Design review of the part built by this model. Coordinates are the model's own, in mm. Face numbers are marked on the shaded views. A direction names the side the tool comes from. Coordinates: 2 decimals unless noted, no trailing zeros. Write each loop counter-clockwise with the first axis right and the second up, starting at its lowest first coordinate (ties: lowest second). Pieces come first, ordered by that corner, then holes. Notation, with made-up numbers: M -18.5,28.5 L 6.5,28.5 A12 cw 6.5,42.5 Z; hole C 25,34 d8. An arc over 180 degrees is marked long. Return JSON: item names as keys, results as strings. Group by question number.
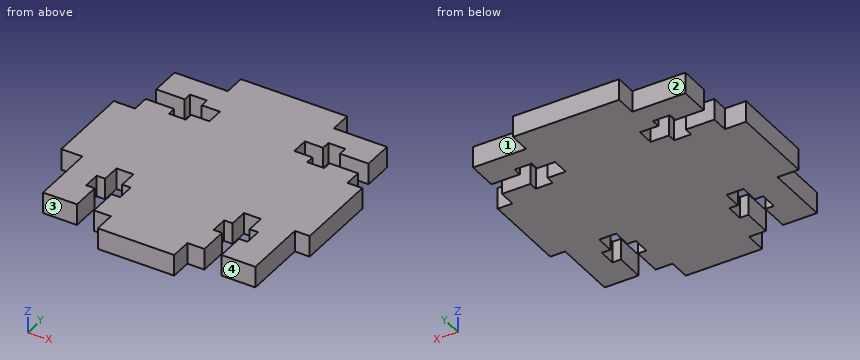
Autodesk Inventor part; units mm, degrees
ref_plane "YZ Plane" through (0, 0, 0) normal (1, 0, 0) x (0, 1, 0)
ref_plane "XZ Plane" through (0, 0, 0) normal (0, 1, 0) x (-1, 0, 0)
ref_plane "XY Plane" through (0, 0, 0) normal (0, 0, 1) x (1, 0, 0)
sketch "Sketch1" plane through (0, 0, 0) normal (0, 0, 1) x (1, 0, 0)
  line L0 (-25, -25) -> (25, -25)
  line L1 (25, -25) -> (25, 25)
  line L2 (25, 25) -> (-25, 25)
  line L3 (-25, 25) -> (-25, -25)
  line L4 (-25, -25) -> (25, 25) construction
  line L5 (25, -25) -> (-25, 25) construction
  point P0 (0, 0)
  dimension "d0" = 50
  dimension "d1" = 50
extrude "Extrusion1" add sketch "Sketch1" along normal blind 5
sketch "Sketch2" plane through (0, 0, 5) normal (0, 0, 1) x (1, 0, 0)
  line L0 (-25, -25) -> (25, -25) construction
  line L1 (25, -25) -> (25, 25) construction
  line L2 (25, 25) -> (-25, 25) construction
  line L3 (-25, 25) -> (-25, -25) construction
  line L4 (-25, -25) -> (25, -25) construction
  line L5 (-9, -25) -> (9, -25)
  line L6 (9, -25) -> (9, -30)
  line L7 (9, -30) -> (-9, -30)
  line L8 (-9, -30) -> (-9, -25)
  line L9 (-25, 10) -> (-30, 10)
  line L10 (-30, 10) -> (-30, -10)
  line L11 (-30, -10) -> (-25, -10)
  line L12 (-25, -10) -> (-25, 10)
  line L13 (25, 25) -> (-25, 25) construction
  line L14 (-12.5, 25) -> (12.5, 25)
  line L15 (12.5, 25) -> (12.5, 30)
  line L16 (12.5, 30) -> (-12.5, 30)
  line L17 (-12.5, 30) -> (-12.5, 25)
  line L18 (25, -10) -> (28.5, -10)
  line L19 (28.5, -10) -> (28.5, 10)
  line L20 (28.5, 10) -> (25, 10)
  line L21 (25, 10) -> (25, -10)
  point P0 (0, 0)
  dimension "d4" = 18
  dimension "d5" = 5
  dimension "d6" = 16
  dimension "d7" = 5
  dimension "d8" = 20
  dimension "d9" = 15
  dimension "d10" = 25
  dimension "d11" = 12.5
  dimension "d14" = 3.5
  dimension "d15" = 20
  dimension "d16" = 15
  dimension "d39" = 5
extrude "Extrusion2" add sketch "Sketch2" against normal blind 5
sketch "Sketch3" plane through (0, 0, 5) normal (0, 0, 1) x (1, 0, 0)
  line L0 (-25, -25) -> (-9, -25) construction
  line L1 (-9, -30) -> (-9, -25) construction
  line L2 (9, -30) -> (-9, -30) construction
  line L3 (9, -25) -> (9, -30) construction
  line L4 (9, -25) -> (25, -25) construction
  line L5 (25, -25) -> (25, -10) construction
  line L6 (25, -10) -> (28.5, -10) construction
  line L7 (28.5, -10) -> (28.5, 10) construction
  line L8 (28.5, 10) -> (25, 10) construction
  line L9 (25, 10) -> (25, 25) construction
  line L10 (25, 25) -> (12.5, 25) construction
  line L11 (12.5, 25) -> (12.5, 30) construction
  line L12 (12.5, 30) -> (-12.5, 30) construction
  line L13 (-12.5, 30) -> (-12.5, 25) construction
  line L14 (-12.5, 25) -> (-25, 25) construction
  line L15 (-25, 25) -> (-25, 10) construction
  line L16 (-25, 10) -> (-30, 10) construction
  line L17 (-30, 10) -> (-30, -10) construction
  line L18 (-30, -10) -> (-25, -10) construction
  line L19 (-25, -10) -> (-25, -25) construction
  line L20 (-25, 25) -> (-25, 10) construction
  line L21 (-25, 18) -> (-10, 18) construction
  line L22 (-10, 18) -> (-10, 14) construction
  line L23 (-10, 14) -> (-25, 14) construction
  line L24 (-25, 14) -> (-25, 18) construction
  line L25 (-10, 16) -> (-25, 16) construction
  line L26 (-18.2831, 12) -> (-14.2831, 12) construction
  line L27 (-14.2831, 12) -> (-14.2831, 20) construction
  line L28 (-14.2831, 20) -> (-18.2831, 20) construction
  line L29 (-18.2831, 20) -> (-18.2831, 12) construction
  line L30 (-18.2831, 12) -> (-14.2831, 20) construction
  line L31 (-14.2831, 12) -> (-18.2831, 20) construction
  line L32 (-25, 14) -> (-25, 18)
  line L33 (-25, 18) -> (-18.2831, 18)
  line L34 (-18.2831, 18) -> (-18.2831, 20)
  line L35 (-18.2831, 20) -> (-14.2831, 20)
  line L36 (-14.2831, 20) -> (-14.2831, 18)
  line L37 (-14.2831, 18) -> (-10, 18)
  line L38 (-10, 18) -> (-10, 14)
  line L39 (-10, 14) -> (-14.2831, 14)
  line L40 (-14.2831, 14) -> (-14.2831, 12)
  line L41 (-14.2831, 12) -> (-18.2831, 12)
  line L42 (-18.2831, 12) -> (-18.2831, 14)
  line L43 (-18.2831, 14) -> (-25, 14)
  line L44 (-17, -25) -> (-17, -10) construction
  line L45 (-17, -10) -> (-13, -10) construction
  line L46 (-13, -10) -> (-13, -25) construction
  line L47 (-13, -25) -> (-17, -25) construction
  line L48 (-15, -10) -> (-15, -25) construction
  line L49 (-11, -18.2831) -> (-11, -14.2831) construction
  line L50 (-11, -14.2831) -> (-19, -14.2831) construction
  line L51 (-19, -14.2831) -> (-19, -18.2831) construction
  line L52 (-19, -18.2831) -> (-11, -18.2831) construction
  line L53 (-11, -18.2831) -> (-19, -14.2831) construction
  line L54 (-11, -14.2831) -> (-19, -18.2831) construction
  line L55 (-13, -25) -> (-17, -25)
  line L56 (-17, -25) -> (-17, -18.2831)
  line L57 (-17, -18.2831) -> (-19, -18.2831)
  line L58 (-19, -18.2831) -> (-19, -14.2831)
  line L59 (-19, -14.2831) -> (-17, -14.2831)
  line L60 (-17, -14.2831) -> (-17, -10)
  line L61 (-17, -10) -> (-13, -10)
  line L62 (-13, -10) -> (-13, -14.2831)
  line L63 (-13, -14.2831) -> (-11, -14.2831)
  line L64 (-11, -14.2831) -> (-11, -18.2831)
  line L65 (-11, -18.2831) -> (-13, -18.2831)
  line L66 (-13, -18.2831) -> (-13, -25)
  line L67 (13, -10) -> (17, -10) construction
  line L68 (13, -10) -> (17, -10)
  line L69 (11, -14.2831) -> (13, -14.2831)
  line L70 (13, -14.2831) -> (13, -10)
  line L71 (17, -10) -> (17, -14.2831)
  line L72 (19, -14.2831) -> (11, -14.2831) construction
  line L73 (17, -14.2831) -> (19, -14.2831)
  line L74 (11, -14.2831) -> (11, -18.2831) construction
  line L75 (11, -18.2831) -> (11, -14.2831)
  line L76 (19, -18.2831) -> (11, -14.2831) construction
  line L77 (19, -14.2831) -> (11, -18.2831) construction
  line L78 (19, -18.2831) -> (19, -14.2831) construction
  line L79 (19, -14.2831) -> (19, -18.2831)
  line L80 (13, -25) -> (13, -10) construction
  line L81 (15, -10) -> (15, -25) construction
  line L82 (17, -10) -> (17, -25) construction
  line L83 (13, -18.2831) -> (11, -18.2831)
  line L84 (19, -18.2831) -> (17, -18.2831)
  line L85 (17, -18.2831) -> (17, -25)
  line L86 (17, -25) -> (13, -25) construction
  line L87 (17, -25) -> (13, -25)
  line L88 (13, -25) -> (13, -18.2831)
  line L89 (11, -18.2831) -> (19, -18.2831) construction
  line L90 (25, 14) -> (10, 14) construction
  line L91 (10, 14) -> (10, 18) construction
  line L92 (10, 18) -> (25, 18) construction
  line L93 (25, 18) -> (25, 14) construction
  line L94 (10, 16) -> (25, 16) construction
  line L95 (18.2831, 20) -> (14.2831, 20) construction
  line L96 (14.2831, 20) -> (14.2831, 12) construction
  line L97 (14.2831, 12) -> (18.2831, 12) construction
  line L98 (18.2831, 12) -> (18.2831, 20) construction
  line L99 (18.2831, 20) -> (14.2831, 12) construction
  line L100 (14.2831, 20) -> (18.2831, 12) construction
  line L101 (25, 18) -> (25, 14)
  line L102 (25, 14) -> (18.2831, 14)
  line L103 (18.2831, 14) -> (18.2831, 12)
  line L104 (18.2831, 12) -> (14.2831, 12)
  line L105 (14.2831, 12) -> (14.2831, 14)
  line L106 (14.2831, 14) -> (10, 14)
  line L107 (10, 14) -> (10, 18)
  line L108 (10, 18) -> (14.2831, 18)
  line L109 (14.2831, 18) -> (14.2831, 20)
  line L110 (14.2831, 20) -> (18.2831, 20)
  line L111 (18.2831, 20) -> (18.2831, 18)
  line L112 (18.2831, 18) -> (25, 18)
  point P0 (0, 0)
  point P1 (-16.2831, 16)
  point P2 (-15, -16.2831)
  point P3 (15, -16.2831)
  point P4 (16.2831, 16)
  dimension "d17" = 15
  dimension "d18" = 4
  dimension "d19" = 4
  dimension "d20" = 8
  dimension "d21" = 15
  dimension "d22" = 4
  dimension "d23" = 4
  dimension "d24" = 8
  dimension "d25" = 15
  dimension "d26" = 4
  dimension "d27" = 4
  dimension "d28" = 8
  dimension "d29" = 8
  dimension "d30" = 4
  dimension "d31" = 4
  dimension "d32" = 15
  dimension "d33" = 4
  dimension "d34" = 4
  dimension "d35" = 8
  dimension "d36" = 7
extrude "Extrusion3" cut sketch "Sketch3" against normal blind 5
properties part number "Soporte_Ducto_Rod"
Item 1: Add section A-A (y = 13). Write out the cut boundary in (x, z).
Item 2: For pin 1 (1 mm diameter, centred on x = 18, z = 3, fed in from +Y); pin 2 (0.6 mm diameter, centred on x = 18, z = 2, fed in from -Y); pin 3 (1.6 mm diameter, centred on y = 12.5, z = 1.5, fed in from +X), all flat-tipped, find the tip position at first contact; note any pin that passes through.
Item 3: For line 1 (X direction, y = -11, z = 4.35); line 2 (Y direction, x = 18.5, z = 4.2); line 3 (Y direction, x = 21.5, z = 0.2), list the stretches that pass through material, from the lowest coordinate up.
Item 4: Add section B-B (y = -17). Write out the cut boundary in (x, z).
Item 5: Machinability: for the marked faces 1, 2, 3 and 4, which of the approach directions +Z, -Z, +X, -X, +Y, -Y give a long, thin tool a straight path to every point of the face, cutting with its end or side? Answer none if there is none.
Geometry check:
{
 "1": {"outline": "M -25,0 L -18.28,0 L -18.28,5 L -25,5 Z; M -14.28,0 L 14.28,0 L 14.28,5 L -14.28,5 Z; M 18.28,0 L 25,0 L 25,5 L 18.28,5 Z"},
 "2": {"pin 1": "y = 25", "pin 2": "y = -25", "pin 3": "x = 25"},
 "3": {"line 1": "-25 to -17, -13 to 13, 17 to 25", "line 2": "-25 to -18.28, -14.28 to 14, 18 to 25", "line 3": "-25 to 14, 18 to 25"},
 "4": {"outline": "M -25,0 L -19,0 L -19,5 L -25,5 Z; M -11,0 L 11,0 L 11,5 L -11,5 Z; M 19,0 L 25,0 L 25,5 L 19,5 Z"},
 "5": {"face 1": "+Z, -Z, +X, +Y", "face 2": "+Z, -Z, -X, +Y", "face 3": "+Z, -Z, -X, -Y", "face 4": "+Z, -Z, +X, -Y"}
}
